Geometry: final body of the model. Coordinates: model frame, mm. A direction names the side the tool comes from. Round coordinates to 2 decimals unless told otherwise and drop trailing zeros. Write each loop counter-clockwise with the first axis right and the second up, starting at its lowest first coordinate (ties: lowest second). Pieces come first, ordered by that corner, then holes. Notation, with made-up numbers: (88, -22.5) - (137, -22.5) arc R24 cw to (137, 2.5) - close; hole circle Ø5 at (47, -16). An arc over 180 degrees is marked (long way). Write each question's results on one line, items separated by ' | '.
from build123d import *

# Parameters (mm, degrees)
EXTRUDE_1_DEPTH          = 1.5
FILLET_1_R               = 2
CUT_EXTRUDE_1_DEPTH      = 48.129161057
CUT_EXTRUDE_1_DEPTH_BACK = 48.129161057
SKETCH_2_R               = 1.25
EXTRUDE_2_DEPTH          = 1.3
SKETCH_5_R               = 0.5
EXTRUDE_3_DEPTH          = 1
CUT_EXTRUDE_2_DEPTH      = 48.161401823
CUT_EXTRUDE_2_DEPTH_BACK = 48.161401823
SKETCH_6_R               = 4
CHAMFER_1_SIZE           = 0.5


with BuildPart() as part:
    # 草图1 → 凸台-拉伸1 (new body)
    with BuildSketch(Plane(origin=(0, 0, 0), x_dir=(1, 0, 0), z_dir=(0, 1, 0))):
        with BuildLine():
            Line((4, 4.472135955), (4, 34.770677301))
            ThreePointArc((4, 34.770677301), (0, 35), (-4, 34.770677301))
            Line((-4, 34.770677301), (-4, 4.472135955))
            ThreePointArc((-4, 4.472135955), (-5.196152423, 3), (-5.872983346, 1.228033638))
            Line((-5.872983346, 1.228033638), (-32.11228985, -13.921237036))
            ThreePointArc((-32.11228985, -13.921237036), (-30.310889132, -17.5), (-28.11228985, -20.849440266))
            Line((-28.11228985, -20.849440266), (-1.872983346, -5.700169593))
            ThreePointArc((-1.872983346, -5.700169593), (0, -6), (1.872983346, -5.700169593))
            Line((1.872983346, -5.700169593), (28.11228985, -20.849440266))
            ThreePointArc((28.11228985, -20.849440266), (30.310889132, -17.5), (32.11228985, -13.921237036))
            Line((32.11228985, -13.921237036), (5.872983346, 1.228033638))
            ThreePointArc((5.872983346, 1.228033638), (5.196152423, 3), (4, 4.472135955))
        make_face()
    extrude(amount=EXTRUDE_1_DEPTH)

    # 圆角1
    fillet_1_edges = [part.edges().sort_by_distance(p)[0] for p in [
        (32.11228985, 0.75, 13.921237036),
        (28.11228985, 0.75, 20.849440266),
        (-28.11228985, 0.75, 20.849440266),
        (-32.11228985, 0.75, 13.921237036),
        (-4, 0.75, -34.770677301),
        (4, 0.75, -34.770677301),
    ]]
    fillet(fillet_1_edges, radius=FILLET_1_R)

    # 草图2 → 切除-拉伸1 (cut, two sides: drawn at the far end of the back side and taken through both)
    with BuildSketch(Plane(origin=(0, 1.5, 0), x_dir=(1, 0, 0), z_dir=(0, 1, 0)).offset(-CUT_EXTRUDE_1_DEPTH_BACK)):
        with Locations(Location((0, 31.5, 0), (0, 0, 270))):
            Circle(SKETCH_2_R)
        with Locations(Location((27.279800219, -15.75, 0), (0, 0, 270))):
            Circle(SKETCH_2_R)
        with Locations(Location((-27.279800219, -15.75, 0), (0, 0, 270))):
            Circle(SKETCH_2_R)
    extrude(amount=CUT_EXTRUDE_1_DEPTH + CUT_EXTRUDE_1_DEPTH_BACK, mode=Mode.SUBTRACT)

    # 草图4 → 凸台-拉伸2 (add)
    with BuildSketch(Plane(origin=(0, 1.5, 0), x_dir=(1, 0, 0), z_dir=(0, 1, 0))):
        with BuildLine():
            Line((-4, 4.472135955), (-4, -4.472135955))
            ThreePointArc((-4, -4.472135955), (-6, 0), (-4, 4.472135955))
        make_face()
        with BuildLine():
            Line((4, 4.472135955), (4, -4.472135955))
            ThreePointArc((4, -4.472135955), (6, 0), (4, 4.472135955))
        make_face()
    extrude(amount=EXTRUDE_2_DEPTH)

    # 草图5 → 凸台-拉伸3 (add)
    with BuildSketch(Plane(origin=(0, 2.8, 0), x_dir=(1, 0, 0), z_dir=(0, 1, 0))):
        with Locations(Location((5, 0, 0), (0, 0, 270))):
            Circle(SKETCH_5_R)
        with Locations(Location((-5, 0, 0), (0, 0, 90))):
            Circle(SKETCH_5_R)
    extrude(amount=EXTRUDE_3_DEPTH)

    # 草图6 → 切除-拉伸2 (cut, two sides: drawn at the far end of the back side and taken through both)
    with BuildSketch(Plane(origin=(0, 1.5, 0), x_dir=(1, 0, 0), z_dir=(0, 1, 0)).offset(-CUT_EXTRUDE_2_DEPTH_BACK)):
        with Locations(Location((0, 0, 0), (0, 0, 270))):
            Circle(SKETCH_6_R)
    extrude(amount=CUT_EXTRUDE_2_DEPTH + CUT_EXTRUDE_2_DEPTH_BACK, mode=Mode.SUBTRACT)

    # 倒角1
    chamfer_1_edges = [part.edges().sort_by_distance(p)[0] for p in [
        (0, 0, 6),
    ]]
    chamfer(chamfer_1_edges, length=CHAMFER_1_SIZE)


solid = part.part
Q1. Section query B-B, the plane z = -28. Return loops of the section in (x, y).
Answer block:
outline: (-4, 0) - (4, 0) - (4, 1.5) - (-4, 1.5) - close
Q2. Pin query (flat end, axial travel): pin 1 (1.6 mm diameter, centred on y = 0.5, z = -12, fed in from -X); pin 2 (1.2 mm diameter, centred on y = 1, z = -14, fed in from +X); pin 3 (23.5 mm diameter, centred on x = -14, z = 11, fed in from +Y). Return the tip coordinate at first contact, or that it passes through.
Answer block:
pin 1: x = -4 | pin 2: x = 4 | pin 3: y = 1.5
Q3. Ray query, line 1 along Z through (x, y) = (0, 0.8); line 2 along X through (y, z) = (0.3, 15.75); line 3 along X through (y, z) = (0.9, -31.5). Return the intervals inside material, ascending.
Answer block:
line 1: -35 to -32.75, -30.25 to -4, 4 to 6 | line 2: -31.26 to -28.53, -26.03 to -19.28, 19.28 to 26.03, 28.53 to 31.26 | line 3: -4 to -1.25, 1.25 to 4
Q4. Section query C-C, the plane x = -7.5. Return loops of the section in (y, z).
Answer block:
outline: (0, -0.29) - (1.5, -0.29) - (1.5, 8.95) - (0, 8.95) - close
Q5. Access query for faces 1 (the cylindrical face through (30.296, 0.74, 17.526)), 2 (the flat face through (-4, 1, -19)), 3 (the flat face through (-4, 2, 0)). Directions: +Z, -Z, +X, -X, +Y, -Y. A direction counts if a zero-diameter tool reaches every point of the face in a straight line with its end or side. Return the directions, or none.
Answer block:
face 1: +Z, +X, +Y, -Y | face 2: -Z, -X, +Y, -Y | face 3: +Z, -Z, +Y
Q6. Section query A-A, the plane x = 0. Return loops of the section in (y, z), plus the area to 3 significant figures.
Answer block:
outline: (0, -35) - (1.5, -35) - (1.5, -32.75) - (0, -32.75) - close; (0, -30.25) - (1.5, -30.25) - (1.5, -4) - (0, -4) - close; (0, 4) - (1.5, 4) - (1.5, 6) - (0.5, 6) - (0, 5.5) - close | area: 45.6 mm2
Q7. Mould query, pull axis Z, two halves, no side actions, for faces 4 (the cylindrical face through (-30.33, 0.74, 17.47)), 5 (the flat face through (4, 1, -19)), 6 (the cylindrical face through (26.06, 0.74, 15.48)). Classes: pulls with the +Z half, pulls with the -Z half, needs draft (parallel to the pull), parting line crosses it, or undercut.
Answer block:
face 4: pulls with the +Z half | face 5: needs draft | face 6: undercut
